from build123d import *

# Parameters (mm, degrees)
BOSS_EXTRUDE1_DEPTH = 3
FILLET1_R           = 2
FILLET2_R           = 0.5


with BuildPart() as part:
    # Sketch1 → Boss-Extrude1 (new body)
    with BuildSketch(Plane(origin=(0, 0, 0), x_dir=(1, 0, 0), z_dir=(0, 1, 0))):
        Polygon((0.555255475, 90.8817274), (16.555255475, 90.8817274), (16.555255475, 95.6317274), (19.555255475, 95.6317274), (19.555255475, 102.8817274), (-2.444744525, 102.8817274), (-2.444744525, 95.6317274), (0.555255475, 95.6317274), align=None)
        with BuildLine():
            ThreePointArc((8.055255475, 100.3817274), (8.555255475, 100.8817274), (9.055255475, 100.3817274))
            Line((9.055255475, 100.3817274), (9.055255475, 93.8817274))
            ThreePointArc((9.055255475, 93.8817274), (8.555255475, 93.3817274), (8.055255475, 93.8817274))
            Line((8.055255475, 93.8817274), (8.055255475, 100.3817274))
        make_face(mode=Mode.SUBTRACT)
    extrude(amount=BOSS_EXTRUDE1_DEPTH)

    # Fillet1
    fillet1_edges = [part.edges().sort_by_distance(p)[0] for p in [
        (-2.444744525, 1.5, -102.8817274),
        (19.555255475, 1.5, -102.8817274),
    ]]
    fillet(fillet1_edges, radius=FILLET1_R)

    # Fillet2
    fillet2_edges = [part.edges().sort_by_distance(p)[0] for p in [
        (-2.444744525, 1.5, -95.6317274),
        (19.555255475, 1.5, -95.6317274),
        (16.555255475, 1.5, -90.8817274),
        (0.555255475, 1.5, -90.8817274),
    ]]
    fillet(fillet2_edges, radius=FILLET2_R)


solid = part.part
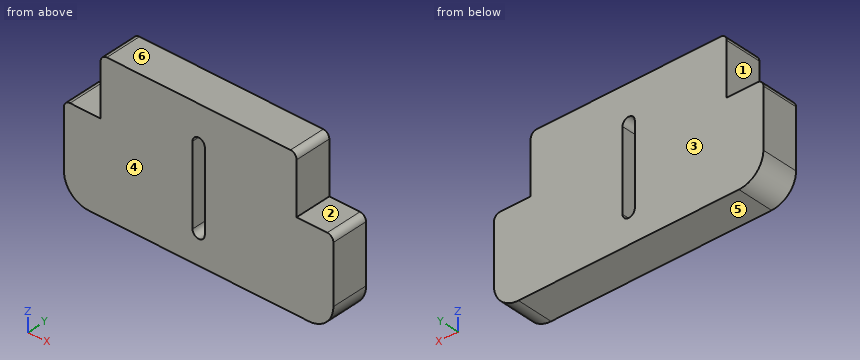
The model under review builds one solid part; all positions refer to its coordinate system, in mm. Face numbers are marked on the shaded views. A direction names the side the tool comes from. Coordinates: 2 decimals unless noted, no trailing zeros. Order: outer loops, then holes, each group sorted by start corner. A loop starts at its lowest first (then second) coordinate and runs counter-clockwise, first axis right, second up. Notation, with made-up numbers: (-11, 8.25) -> (23, 8.25) arc R20 ccw to (23, 12.25) -> close; hole circle Ø9 at (8, 71). An arc over 180 degrees is marked (long way). Answer in a Markdown table with one row per item.
(1) Consider section C-C (x = 8.75). Write out the cut boundary in (y, z).
Answers:
| item | result |
|---|---|
| outline | (0, -102.88) -> (3, -102.88) -> (3, -100.84) -> (0, -100.84) -> close; (0, -93.42) -> (3, -93.42) -> (3, -90.88) -> (0, -90.88) -> close |
(2) Consider section B-B (z = -97). Write out the cut boundary in (x, y).
Answers:
| item | result |
|---|---|
| outline | (-2.44, 0) -> (8.06, 0) -> (8.06, 3) -> (-2.44, 3) -> close; (9.06, 0) -> (19.56, 0) -> (19.56, 3) -> (9.06, 3) -> close |
(3) Machinability: for the marked faces 1, 2 and 3, which of the approach directions +Z, -Z, +X, -X, +Y, -Y give a long, thin tool a straight path to every point of the face, cutting with its end or side? Answer none if there is none.
Answers:
| item | result |
|---|---|
| face 1 | +Z, -X, +Y, -Y |
| face 2 | +Z, +X, +Y, -Y |
| face 3 | +Z, -Z, +X, -X, +Y |
(4) Wall thickness on line 1 along Z through (x, y) = (8.5, 1.7); line 2 along X through (y, z) = (1.6, -96.25); line 3 along X through (y, z) = (1.75, -95.25): over which ranges is each line inside the solid? List them lowest first.
Answers:
| item | result |
|---|---|
| line 1 | -102.88 to -100.88, -93.38 to -90.88 |
| line 2 | -2.44 to 8.06, 9.06 to 19.56 |
| line 3 | 0.56 to 8.06, 9.06 to 16.56 |
(5) Consider section D-D (z = -91.75). Write out the cut boundary in (x, y), plus the area to 3 significant figures.
Answers:
| item | result |
|---|---|
| outline | (0.56, 0) -> (16.56, 0) -> (16.56, 3) -> (0.56, 3) -> close |
| area | 48.0 mm² |
(6) The part is to be moulded in two halves that separate along Z. For the marked faces 4, 5 and 6, say which applies: +Z half, -Z half, draft (parallel to the pull), parting line (faces both ways), or undercut.
Answers:
| item | result |
|---|---|
| face 4 | draft |
| face 5 | -Z half |
| face 6 | +Z half |
(7) Consider section A-A (y = 1.15). Write out the cut boundary in (x, z), plus the area to 3 significant figures.
Answers:
| item | result |
|---|---|
| outline | (-2.44, -100.88) arc R2 ccw to (-0.44, -102.88) -> (17.56, -102.88) arc R2 ccw to (19.56, -100.88) -> (19.56, -96.13) arc R0.5 ccw to (19.06, -95.63) -> (16.56, -95.63) -> (16.56, -91.38) arc R0.5 ccw to (16.06, -90.88) -> (1.06, -90.88) arc R0.5 ccw to (0.56, -91.38) -> (0.56, -95.63) -> (-1.94, -95.63) arc R0.5 ccw to (-2.44, -96.13) -> close; hole (8.06, -100.38) arc R0.5 ccw to (9.06, -100.38) -> (9.06, -93.88) arc R0.5 ccw to (8.06, -93.88) -> close |
| area | 226 mm² |
